The listing builds one solid part. Answer for the finished solid, in the listing's coordinates (mm). Coordinates: 2 decimals unless noted, no trailing zeros. Write each loop counter-clockwise with the first axis right and the second up, starting at its lowest first coordinate (ties: lowest second). Pieces come first, ordered by that corner, then holes. Notation, with made-up numbers: M -12.5,26.5 L -3.5,26.5 A6 cw -3.5,34.5 Z; hole C 44.5,54.25 d3. An arc over 180 degrees is marked long. Answer as CSV lines item,"result".
```python
from build123d import *

# Parameters (mm, degrees)
SKETCH_1_W          = 15
SKETCH_1_H          = 15
EXTRUDE_1_DEPTH     = 20
SKETCH_2_R          = 2.45
CUT_EXTRUDE_1_DEPTH = 16
SKETCH_3_R          = 2.45
CUT_EXTRUDE_2_DEPTH = 16
FILLET_1_R          = 2
CHAMFER_1_SIZE      = 1


with BuildPart() as part:
    # ｽｹｯﾁ1 → ﾎﾞｽ - 押し出し1 (new body)
    with BuildSketch(Plane.XY):
        Rectangle(SKETCH_1_W, SKETCH_1_H)
    extrude(amount=EXTRUDE_1_DEPTH)

    # ｽｹｯﾁ2 → ｶｯﾄ - 押し出し1 (cut, through all)
    with BuildSketch(Plane(origin=(7.5, 0, 0), x_dir=(0, 0, -1), z_dir=(1, 0, 0))):
        with Locations((-5, 0)):
            Circle(SKETCH_2_R)
    extrude(amount=-CUT_EXTRUDE_1_DEPTH, mode=Mode.SUBTRACT)

    # ｽｹｯﾁ3 → ｶｯﾄ - 押し出し2 (cut, through all)
    with BuildSketch(Plane(origin=(0, 7.5, 0), x_dir=(1, 0, 0), z_dir=(0, 1, 0))):
        with Locations((0, -15)):
            Circle(SKETCH_3_R)
    extrude(amount=-CUT_EXTRUDE_2_DEPTH, mode=Mode.SUBTRACT)

    # ﾌｨﾚｯﾄ1
    fillet_1_edges = [part.edges().sort_by_distance(p)[0] for p in [
        (7.5, -7.5, 10),
        (-7.5, -7.5, 10),
        (-7.5, 7.5, 10),
        (7.5, 7.5, 10),
    ]]
    fillet(fillet_1_edges, radius=FILLET_1_R)

    # 面取り1
    chamfer_1_edges = [part.edges().sort_by_distance(p)[0] for p in [
        (7.5, 0, 0),
        (7.5, 0, 20),
        (0, -7.5, 0),
        (-7.5, 0, 0),
        (0, 7.5, 0),
        (6.914213562, 6.914213562, 0),
        (-6.914213562, 6.914213562, 0),
        (-6.914213562, -6.914213562, 0),
        (6.914213562, -6.914213562, 0),
        (0, -7.5, 20),
        (0, 7.5, 20),
        (-7.5, 0, 20),
        (6.914213562, 6.914213562, 20),
        (-6.914213562, 6.914213562, 20),
        (-6.914213562, -6.914213562, 20),
        (6.914213562, -6.914213562, 20),
    ]]
    chamfer(chamfer_1_edges, length=CHAMFER_1_SIZE)


solid = part.part
```
Q1. Find section B-B (z = 5). Give the vertices of the cut face in (x, y), and give its area (3 significant figures).
Output:
outline,"M -7.5,-5.5 A2 ccw -5.5,-7.5 L 5.5,-7.5 A2 ccw 7.5,-5.5 L 7.5,-2.45 L -7.5,-2.45 Z; M -7.5,2.45 L 7.5,2.45 L 7.5,5.5 A2 ccw 5.5,7.5 L -5.5,7.5 A2 ccw -7.5,5.5 Z"
area,"148 mm2"
Q2. Find section D-D (x = -3.5). Give the vertices of the cut face in (y, z), and give its area (3 significant figures).
Output:
outline,"M -7.5,1 L -6.5,0 L 6.5,0 L 7.5,1 L 7.5,19 L 6.5,20 L -6.5,20 L -7.5,19 Z; hole C 0,5 d4.9"
area,"279 mm2"
Q3. Find section A-A (y = 0). Give the vertices of the cut face in (x, z), and give its area (3 significant figures).
Output:
outline,"M -7.5,1 L -6.5,0 L 6.5,0 L 7.5,1 L 7.5,2.55 L -7.5,2.55 Z; M -7.5,7.45 L 7.5,7.45 L 7.5,19 L 6.5,20 L -6.5,20 L -7.5,19 Z; hole C 0,15 d4.9"
area,"206 mm2"
Q4. Find section C-C (x = 0). Give the vertices of the cut face in (y, z).
Output:
outline,"M -7.5,1 L -6.5,0 L 6.5,0 L 7.5,1 L 7.5,12.55 L -7.5,12.55 Z; M -7.5,17.45 L 7.5,17.45 L 7.5,19 L 6.5,20 L -6.5,20 L -7.5,19 Z; hole C 0,5 d4.9"
Q5. Straight lines are drawn through the part: line 1 (Y direction, x = -0.25, z = 5); line 2 (Z direction, x = 0, y = 3.25); line 3 (Z direction, x = 0, y = -1.5). For each, find the intervals that lie inside material, in ascending order.
Output:
line 1,"-7.5 to -2.45, 2.45 to 7.5"
line 2,"0 to 12.55, 17.45 to 20"
line 3,"0 to 3.06, 6.94 to 12.55, 17.45 to 20"
Q6. The mould has two halves that part along X. Classify faces 1 (the flat face through (0, 0, 0)), 2 (the cylindrical face through (-0.5, 0.1, 17.4)), 3 (the cylindrical face through (6.9, -6.93, 10.13)): pulls with the +X half, pulls with the -X half, needs draft (parallel to the pull), parting line crosses it, or undercut.
Output:
face 1,"needs draft"
face 2,"undercut"
face 3,"pulls with the +X half"
